```python
from build123d import *

# Parameters (mm, degrees)
SKETCH1_R           = 7.5
SKETCH1_R_2         = 1.5875
BOSS_EXTRUDE1_DEPTH = 20
SKETCH2_R           = 10.5
SKETCH2_R_2         = 7.5
SKETCH2_R_3         = 1.5875
BOSS_EXTRUDE2_DEPTH = 2
SKETCH3_R           = 1
CUT_EXTRUDE1_DEPTH  = 3
SKETCH4_R           = 7.5
SKETCH4_R_2         = 5.5
CUT_EXTRUDE2_DEPTH  = 13
SKETCH5_R           = 5.5
SKETCH5_R_2         = 3.5
CUT_EXTRUDE3_DEPTH  = 8


with BuildPart() as part:
    # Sketch1 → Boss-Extrude1 (new body)
    with BuildSketch(Plane.XY):
        Circle(SKETCH1_R)
        Circle(SKETCH1_R_2, mode=Mode.SUBTRACT)
    extrude(amount=BOSS_EXTRUDE1_DEPTH)

    # Sketch2 → Boss-Extrude2 (add)
    with BuildSketch(Plane.XY.offset(20)):
        Circle(SKETCH2_R)
        Circle(SKETCH2_R_2, mode=Mode.SUBTRACT)
        Circle(SKETCH2_R_2)
        Circle(SKETCH2_R_3, mode=Mode.SUBTRACT)
    extrude(amount=-BOSS_EXTRUDE2_DEPTH)

    # Sketch3 → Cut-Extrude1 (cut, through all)
    with BuildSketch(Plane(origin=(0, 0, 18), x_dir=(-1, 0, 0), z_dir=(0, 0, -1))):
        with Locations((0, 9)):
            Circle(SKETCH3_R)
    extrude(amount=-CUT_EXTRUDE1_DEPTH, mode=Mode.SUBTRACT)

    # Sketch4 → Cut-Extrude2 (cut)
    with BuildSketch(Plane(origin=(0, 0, 0), x_dir=(-1, 0, 0), z_dir=(0, 0, -1))):
        Circle(SKETCH4_R)
        Circle(SKETCH4_R_2, mode=Mode.SUBTRACT)
    extrude(amount=-CUT_EXTRUDE2_DEPTH, mode=Mode.SUBTRACT)

    # Sketch5 → Cut-Extrude3 (cut)
    with BuildSketch(Plane(origin=(0, 0, 0), x_dir=(-1, 0, 0), z_dir=(0, 0, -1))):
        Circle(SKETCH5_R)
        Circle(SKETCH5_R_2, mode=Mode.SUBTRACT)
    extrude(amount=-CUT_EXTRUDE3_DEPTH, mode=Mode.SUBTRACT)


solid = part.part
```
CAD build for the part. Positions are in the model's coordinates, mm. A direction names the side the tool comes from. Round coordinates to 2 decimals unless told otherwise and drop trailing zeros. Order: outer loops, then holes, each group sorted by start corner. A loop starts at its lowest first (then second) coordinate and runs counter-clockwise, first axis right, second up. Notation, with made-up numbers: (58.25, 79) - (108.25, 79) arc R32 ccw to (108.25, 106) - close; hole circle Ø5 at (47, 77.5). An arc over 180 degrees is marked (long way). Use CSV: the item, a comma, the result in double quotes. Start each with the question number.
1) Saw through at B-B (x = 0). List the corners of the cut face in (y, z).
2) Wall check: L1, parallel to Y at x = 0, z = 19.45; L2, parallel to Y at x = 0, z = 5.5; L3, parallel to Y at x = 0, z = 11.5. Give the ranges that are in metal, low to high. Write a range as [from, to].
3) Saw through at A-A (y = 0). List the corners of the cut face in (x, z).
4) Tool access for faces 5 (the flat face through (-4, 0, 8)), 6 (the flat face through (0, -2, 20)): list every direction of +Z, -Z, +X, -X, +Y, -Y with a clear straight run to the whole face (end or side of a thin tool).
5) Pin check, flat tips, straight feed: pin 1 Ø12 at (y, z) = (-7, 16) entering from +X; pin 2 Ø8 at (x, z) = (-2.5, 4.5) entering from +Y; pin 3 Ø1.5 at (y, z) = (0.5, 5) entering from -X. Stop position of each tip, or through.
6) Saw through at D-D (y = -6.5). List the corners of the cut face in (x, z), and give its area (3 significant figures).
7) Two-plate mould, pull along X, no slides. Class faces 1 (the cylindrical face through (10, 3.2, 19)), 2 (the cylindrical face through (0, 10, 19)), 3 (the flat face through (4, 4, 13)), 4 (the cylindrical face through (-0.34, -1.55, 9.86)): pulls with the +X half, pulls with the -X half, needs draft (parallel to the pull), parting line crosses it, or undercut.
8) Saw through at C-C (z = 11.25). List the corners of the cut face in (x, y) (1 decimal), and give its area (3 significant figures).
Values follow:
1,outline,"(-10.5, 18) - (-7.5, 18) - (-7.5, 13) - (-5.5, 13) - (-5.5, 8) - (-3.5, 8) - (-3.5, 0) - (-1.59, 0) - (-1.59, 20) - (-10.5, 20) - close; (1.59, 0) - (3.5, 0) - (3.5, 8) - (5.5, 8) - (5.5, 13) - (7.5, 13) - (7.5, 18) - (8, 18) - (8, 20) - (1.59, 20) - close; (10, 18) - (10.5, 18) - (10.5, 20) - (10, 20) - close"
2,L1,"y = [-10.5, -1.59], [1.59, 8], [10, 10.5]"
2,L2,"y = [-3.5, -1.59], [1.59, 3.5]"
2,L3,"y = [-5.5, -1.59], [1.59, 5.5]"
3,outline,"(-10.5, 18) - (-7.5, 18) - (-7.5, 13) - (-5.5, 13) - (-5.5, 8) - (-3.5, 8) - (-3.5, 0) - (-1.59, 0) - (-1.59, 20) - (-10.5, 20) - close; (1.59, 0) - (3.5, 0) - (3.5, 8) - (5.5, 8) - (5.5, 13) - (7.5, 13) - (7.5, 18) - (10.5, 18) - (10.5, 20) - (1.59, 20) - close"
4,face 5,"-Z"
4,face 6,"+Z, +X, -X, +Y, -Y"
5,pin 1,"stops at x = 10.41"
5,pin 2,"stops at y = 5.47"
5,pin 3,"stops at x = -3.5"
6,outline,"(-8.25, 18) - (-3.74, 18) - (-3.74, 13) - (3.74, 13) - (3.74, 18) - (8.25, 18) - (8.25, 20) - (-8.25, 20) - close"
6,area,"70.4 mm2"
7,face 1,"parting line crosses it"
7,face 2,"undercut"
7,face 3,"needs draft"
7,face 4,"undercut"
8,outline,"circle Ø11 at (0, 0); hole circle Ø3.2 at (0, 0)"
8,area,"87.1 mm2"
